from build123d import *

# Parameters (mm, degrees)
F0_W     = 25
F0_H     = 25
F1_DEPTH = 6
F2_W     = 21
F2_H     = 21
F2_W_2   = 11
F2_H_2   = 11
F2_W_3   = 5
F2_H_3   = 5
F3_DEPTH = 2.7
F4_START = 3.5
F4_DEPTH = 2.501
F5_SIZE  = 0.6
F6_SIZE2 = 2.69999
F6_SIZE  = 0.99999


# Not quite as in the source:
# - a fillet or chamfer is up to 0.001 mm smaller than in the source, because OpenCascade refuses the exact size


with BuildPart() as f1:
    # F0 (on Top) → F1 (new body)
    with BuildSketch(Plane.XY):
        Rectangle(F0_W, F0_H)
        Polygon((-7.4246212025, 7.4246212025), (-2.0710678119, 5), (0, 10.5), (2.0710678119, 5), (7.4246212025, 7.4246212025), (5, 2.0710678119), (10.5, 0), (5, -2.0710678119), (7.4246212025, -7.4246212025), (2.0710678119, -5), (0, -10.5), (-2.0710678119, -5), (-7.4246212025, -7.4246212025), (-5, -2.0710678119), (-10.5, 0), (-5, 2.0710678119), align=None, mode=Mode.SUBTRACT)
        Polygon((0, 10.5), (-2.0710678119, 5), (-7.4246212025, 7.4246212025), (-5, 2.0710678119), (-10.5, 0), (-5, -2.0710678119), (-7.4246212025, -7.4246212025), (-2.0710678119, -5), (0, -10.5), (2.0710678119, -5), (7.4246212025, -7.4246212025), (5, -2.0710678119), (10.5, 0), (5, 2.0710678119), (7.4246212025, 7.4246212025), (2.0710678119, 5), align=None)
    extrude(amount=F1_DEPTH)

    # F2 (on Top) → F3 (cut)
    with BuildSketch(Plane.XY):
        Rectangle(F2_W, F2_H)
        Rectangle(F2_W_2, F2_H_2, mode=Mode.SUBTRACT)
        Rectangle(F2_W_3, F2_H_3)
    extrude(amount=F3_DEPTH, mode=Mode.SUBTRACT)

    # F0 (on Top) → F4 (cut)
    with BuildSketch(Plane.XY.offset(F4_START)):
        Polygon((0, 10.5), (-2.0710678119, 5), (-7.4246212025, 7.4246212025), (-5, 2.0710678119), (-10.5, 0), (-5, -2.0710678119), (-7.4246212025, -7.4246212025), (-2.0710678119, -5), (0, -10.5), (2.0710678119, -5), (7.4246212025, -7.4246212025), (5, -2.0710678119), (10.5, 0), (5, 2.0710678119), (7.4246212025, 7.4246212025), (2.0710678119, 5), align=None)
    extrude(amount=F4_DEPTH, mode=Mode.SUBTRACT)

    # F5
    f5_edges = [f1.edges().sort_by_distance(p)[0] for p in [
        (0, -12.5, 6),
        (-12.5, -12.5, 3),
        (-12.5, 0, 6),
        (-12.5, 12.5, 3),
        (0, 12.5, 6),
        (12.5, 0, 6),
        (12.5, -12.5, 3),
        (12.5, 12.5, 3),
        (0, -12.5, 0),
        (12.5, 0, 0),
        (0, 12.5, 0),
        (-12.5, 0, 0),
    ]]
    chamfer(f5_edges, length=F5_SIZE)

    # F6 (size 1 and 2.7 in the source; OpenCascade refuses exactly that, so slightly less here)
    f6_edges = [f1.edges().sort_by_distance(p)[0] for p in [
        (-5.5, 0, 0),
        (0, 5.5, 0),
        (5.5, 0, 0),
        (0, -5.5, 0),
        (-2.5, 0, 0),
        (0, -2.5, 0),
        (2.5, 0, 0),
        (0, 2.5, 0),
    ]]
    f6_side = f1.faces().sort_by_distance((-5.344437, 0, 0))[0]
    chamfer(f6_edges, length=F6_SIZE, length2=F6_SIZE2, reference=f6_side)


solid = f1.part
Here's how the part is built. I have some questions about the finished solid (model axes, mm). A direction names the side the tool comes from. Coordinates: 2 decimals unless noted, no trailing zeros. Order: outer loops, then holes, each group sorted by start corner. A loop starts at its lowest first (then second) coordinate and runs counter-clockwise, first axis right, second up. Notation, with made-up numbers: (-21, 61) -> (-17, 61) arc R9 cw to (-17, 74) -> close; hole circle Ø4 at (6.25, -36.5). An arc over 180 degrees is marked (long way). Answer in a Markdown table with one row per item.
(1) Please list where these lines run through material, in increasing order: probe 1 along X at (y, z) = (-7.25, 1.75); probe 2 along X at (y, z) = (-1, 2.5); probe 3 along X at (y, z) = (-3.25, 1.75).
Answer key:
| item | result |
|---|---|
| probe 1 | -12.5 to -10.5, 10.5 to 12.5 |
| probe 2 | -12.5 to -10.5, -5.43 to -2.57, 2.57 to 5.43, 10.5 to 12.5 |
| probe 3 | -12.5 to -10.5, -5.15 to 5.15, 10.5 to 12.5 |
(2) Will these pins go through, and if not, where does the flat tip stop? pin 1 Ø2.5 at (x, y) = (0, -0.5) entering from -Z; pin 2 Ø2 at (x, z) = (1, 0.5) entering from -Y.
Answer key:
| item | result |
|---|---|
| pin 1 | z = 2.7 |
| pin 2 | y = -12.5 |
(3) Thinking about a two-plate mould opening in X: for faces 3 (the face through (-11, 0, 0)), 4 (the face through (4.79, 6.23, 4.73)), 5 (the face through (-12.5, 0, 3)), which applies, +X half, -X half, draft (parallel to the pull), parting line (faces both ways), or undercut?
Answer key:
| item | result |
|---|---|
| face 3 | draft |
| face 4 | undercut |
| face 5 | -X half |
(4) On a 3-axis mill with a long thin cutter (end or side, diameter ignored), from which of +Z, -Z, +X, -X, +Y, -Y can I reach the whole of each face in a straight line? I mean faces 1 (the face through (6.195, 4.71, 4.732)), 2 (the face through (0, -10.5, 1)). Say none if no direction works.
Answer key:
| item | result |
|---|---|
| face 1 | +Z |
| face 2 | -Z |
(5) I want a section at B-B on z = 4.5. List the corners of the cut face in (x, y) for me, then the cut area to 3 significant figures.
Answer key:
| item | result |
|---|---|
| outline | (-12.5, -11.9) -> (-11.9, -12.5) -> (11.9, -12.5) -> (12.5, -11.9) -> (12.5, 11.9) -> (11.9, 12.5) -> (-11.9, 12.5) -> (-12.5, 11.9) -> close; hole (-10.5, 0) -> (-5, -2.07) -> (-7.42, -7.42) -> (-2.07, -5) -> (0, -10.5) -> (2.07, -5) -> (7.42, -7.42) -> (5, -2.07) -> (10.5, 0) -> (5, 2.07) -> (7.42, 7.42) -> (2.07, 5) -> (0, 10.5) -> (-2.07, 5) -> (-7.42, 7.42) -> (-5, 2.07) -> close |
| area | 450 mm^2 |
(6) I want a section at C-C on x = 10. List the corners of the cut face in (y, z) for me, then the cut area to 3 significant figures.
Answer key:
| item | result |
|---|---|
| outline | (-12.5, 0.6) -> (-11.9, 0) -> (-10.5, 0) -> (-10.5, 2.7) -> (10.5, 2.7) -> (10.5, 0) -> (11.9, 0) -> (12.5, 0.6) -> (12.5, 5.4) -> (11.9, 6) -> (0.19, 6) -> (0.19, 3.5) -> (-0.19, 3.5) -> (-0.19, 6) -> (-11.9, 6) -> (-12.5, 5.4) -> close |
| area | 91.6 mm^2 |
(7) I want a section at A-A on z = 1.5. List the corners of the cut face in (x, y) for me, then the cut area to 3 significant figures.
Answer key:
| item | result |
|---|---|
| outline | (-12.5, -11.9) -> (-11.9, -12.5) -> (11.9, -12.5) -> (12.5, -11.9) -> (12.5, 11.9) -> (11.9, 12.5) -> (-11.9, 12.5) -> (-12.5, 11.9) -> close; (-5.06, -5.06) -> (5.06, -5.06) -> (5.06, 5.06) -> (-5.06, 5.06) -> close; hole (-10.5, -10.5) -> (10.5, -10.5) -> (10.5, 10.5) -> (-10.5, 10.5) -> close; hole (-2.94, -2.94) -> (2.94, -2.94) -> (2.94, 2.94) -> (-2.94, 2.94) -> close |
| area | 251 mm^2 |
(8) I want a section at D-D on y = -8.5. List the corners of the cut face in (x, z) for me.
Answer key:
| item | result |
|---|---|
| outline | (-12.5, 0.6) -> (-11.9, 0) -> (-10.5, 0) -> (-10.5, 2.7) -> (10.5, 2.7) -> (10.5, 0) -> (11.9, 0) -> (12.5, 0.6) -> (12.5, 5.4) -> (11.9, 6) -> (0.75, 6) -> (0.75, 3.5) -> (-0.75, 3.5) -> (-0.75, 6) -> (-11.9, 6) -> (-12.5, 5.4) -> close |
